```python
from build123d import *

# Parameters (mm, degrees)
SKETCH_1_R          = 10
EXTRUDE_1_DEPTH     = 30
CUT_EXTRUDE_1_DEPTH = 30
SKETCH_3_R          = 1
EXTRUDE_2_DEPTH     = 8


with BuildPart() as part:
    # 草图1 → 凸台-拉伸1 (new body)
    with BuildSketch(Plane.XY):
        Circle(SKETCH_1_R)
    extrude(amount=EXTRUDE_1_DEPTH)

    # 草图2 → 切除-拉伸1 (cut)
    with BuildSketch(Plane.XY.offset(30)):
        with BuildLine():
            ThreePointArc((10, 0), (9.354143467, 3.535533906), (7.5, 6.614378278))
            Line((7.5, 6.614378278), (7.5, -6.614378278))
            ThreePointArc((7.5, -6.614378278), (9.354143467, -3.535533906), (10, 0))
        make_face()
        with BuildLine():
            Line((-7.5, -6.614378278), (-7.5, 6.614378278))
            ThreePointArc((-7.5, 6.614378278), (-10, 0), (-7.5, -6.614378278))
        make_face()
    extrude(amount=-CUT_EXTRUDE_1_DEPTH, mode=Mode.SUBTRACT)

    # 草图3 → 凸台-拉伸2 (add)
    with BuildSketch(Plane.XY.offset(30)):
        Circle(SKETCH_3_R)
    extrude(amount=EXTRUDE_2_DEPTH)


solid = part.part
```
Model file for the job. Use its own axes, mm. A direction names the side the tool comes from. Give positions to 0.01 mm unless a question says otherwise; leave off trailing zeros. Loops run counter-clockwise (first coordinate to the right, second up) from the corner with the lowest first, then second, coordinate; pieces in that order, holes last. Notation, with made-up numbers: (83, -17) -> (127, -17) arc R6 cw to (127, -9) -> close; hole circle Ø7 at (29.5, -28). An arc over 180 degrees is marked (long way). Use CSV: the item, a comma, the result in double quotes. Start each with the question number.
1) Slice it at D-D on x = 4. Give the cut face in (y, z).
2) Slice it at C-C on z = 23. Give the cut face in (x, y), plus the area to 3 significant figures.
3) Wall check: line 1 (Z direction, x = -3.5, y = -8.25); line 2 (Y direction, x = 0, z = 18.5); line 3 (Y direction, x = -1.75, z = 29). Give the ranges that are in metal, low to high.
4) Slice it at B-B on x = 0. Give the cut face in (y, z), plus the area to 3 significant figures.
5) Slice it at A-A on y = 0. Give the cut face in (x, z).
6) Tool access for faces 1 (the flat face through (7.5, 0, 15)), 2 (the cylindrical face through (0, -1, 34)): list every direction of +Z, -Z, +X, -X, +Y, -Y with a clear straight run to the whole face (end or side of a thin tool).
7) Flat gauge pins, fed straight in: pin 1 Ø4 at (x, y) = (-1.5, 4.5) entering from +Z; pin 2 Ø1.5 at (y, z) = (-7.5, 21.5) entering from +X; pin 3 Ø5 at (x, z) = (4.5, 21) entering from +Y. Where does each tip first touch, or does it go through?
Computed values:
1,outline,"(-9.17, 0) -> (9.17, 0) -> (9.17, 30) -> (-9.17, 30) -> close"
2,outline,"(-7.5, -6.61) arc R10 ccw to (7.5, -6.61) -> (7.5, 6.61) arc R10 ccw to (-7.5, 6.61) -> close"
2,area,"269 mm^2"
3,line 1,"z = 0 to 30"
3,line 2,"y = -10 to 10"
3,line 3,"y = -9.85 to 9.85"
4,outline,"(-10, 0) -> (10, 0) -> (10, 30) -> (1, 30) -> (1, 38) -> (-1, 38) -> (-1, 30) -> (-10, 30) -> close"
4,area,"616 mm^2"
5,outline,"(-7.5, 0) -> (7.5, 0) -> (7.5, 30) -> (1, 30) -> (1, 38) -> (-1, 38) -> (-1, 30) -> (-7.5, 30) -> close"
6,face 1,"+Z, -Z, +X, +Y, -Y"
6,face 2,"+Z"
7,pin 1,"stops at z = 30"
7,pin 2,"stops at x = 7.38"
7,pin 3,"stops at y = 9.8"
